```python
from build123d import *

# Parameters (mm, degrees)
F0_W     = 40
F0_H     = 40
F1_DEPTH = 40
F4_DEPTH = 30


with BuildPart() as f1:
    # F0 (on Top) → F1 (new body)
    with BuildSketch(Plane.XY):
        Rectangle(F0_W, F0_H)
    extrude(amount=F1_DEPTH)

    # F3 (on 3pt) → F4 (cut, symmetric)
    with BuildSketch(Plane(origin=(0, 0, 0), x_dir=(0.7071067812, 0.7071067812, 0), z_dir=(0.7071067812, -0.7071067812, 0))):
        Polygon((-28.2842712475, 40), (-28.2842712475, 20), (-17.6776695297, 20), (-21.2132034356, 15), (-7.0710678119, 15), (-10.6066017178, 20), (10.6066017178, 20), (7.0710678119, 15), (21.2132034356, 15), (17.6776695297, 20), (28.2842712475, 20), (28.2842712475, 40), align=None)
    extrude(amount=F4_DEPTH, both=True, mode=Mode.SUBTRACT)


solid = f1.part
```
Work out the finished part from the listing and answer in its coordinate system (mm). A direction names the side the tool comes from. Give positions to 0.01 mm unless a question says otherwise; leave off trailing zeros. Order: outer loops, then holes, each group sorted by start corner. A loop starts at its lowest first (then second) coordinate and runs counter-clockwise, first axis right, second up. Notation, with made-up numbers: (-16.75, 43.5) - (3.25, 43.5) arc R19 cw to (3.25, 47.5) - close; hole circle Ø9 at (-12.75, 14). An arc over 180 degrees is marked (long way). One line per item, written item: value. Start each with the question number.
1. Section D-D, the plane y = 14.5 is taken. Write down the section's boundary in (x, z), then the cut area to 3 significant figures.
2. Consider line 1 (X direction, y = 11, z = 15.5); line 2 (Y direction, x = 11, z = 18.5); line 3 (Z direction, x = -2, y = 16). Determine where each line is inside the solid, lowest interval first.
3. Each of these flat-tipped pins is pushed along its axis until it touches: pin 1 Ø3 at (x, y) = (-14.5, 3.5) entering from -Z; pin 2 Ø1 at (x, z) = (3, 17) entering from +Y. Where does it stop, or does it pass through?
4. For a pull along Y with two mould halves and no side action, classify faces 1 (the face through (-15, -16, 20)), 2 (the face through (-6, -6, 17)), 3 (the face through (0, -20, 10)) as released by +Y, released by -Y, zero draft, split by the parting line, or undercut.
5. Section B-B, the plane x = -9 is taken. Write down the section's boundary in (y, z).
6. Section A-A, the plane z = 16.75 is taken. Write down the section's boundary in (x, y), then the cut area to 3 significant figures.
7. Which of the six approach directions +Z, -Z, +X, -X, +Y, -Y give full straight-line access (tool end or side, diameter ignored) to faces 4 (the face through (9, 9, 15)), 5 (the face through (0, 0, 0))?
8. Section C-C, the plane y = -7 is taken. Write down the section's boundary in (x, z), then the cut area to 3 significant figures.
Filled sheet:
1. outline: (-20, 0) - (20, 0) - (20, 20) - (10.5, 20) - (15.5, 15) - (-4.5, 15) - (0.5, 20) - (-20, 20) - close
1. area: 725 mm²
2. line 1: -20 to -0.5, 18.5 to 20
2. line 2: -20 to 2.5, 15.5 to 20
2. line 3: 0 to 15, 19 to 20
3. pin 1: z = 0
3. pin 2: y = 9.71
4. face 1: zero draft
4. face 2: undercut
4. face 3: released by -Y
5. outline: (-20, 0) - (20, 0) - (20, 15) - (19, 15) - (20, 16) - (20, 20) - (-6, 20) - (-1, 15) - (-20, 15) - close; (-20, 16) - (-16, 20) - (-20, 20) - close
6. outline: (-20, -20) - (-8.25, -20) - (-20, -8.25) - close; (-20, 8.25) - (8.25, -20) - (20, -20) - (20, -8.25) - (-8.25, 20) - (-20, 20) - close; (8.25, 20) - (20, 8.25) - (20, 20) - close
6. area: 940 mm²
7. face 4: none
7. face 5: -Z, +X, -X, +Y, -Y
8. outline: (-20, 0) - (20, 0) - (20, 15) - (17, 15) - (20, 18) - (20, 20) - (-8, 20) - (-3, 15) - (-20, 15) - close; (-20, 18) - (-18, 20) - (-20, 20) - close
8. area: 725 mm²
